Autodesk Fusion 360 part; units mm, degrees
sketch "Sketch4" plane through (0, 0, 0) normal (0, 0, 1) x (1, 0, 0)
  line L0 (53.2905, 24.45) -> (-53.2905, 24.45)
  line L1 (-53.2905, 24.45) -> (-53.2905, -24.45)
  line L2 (-53.2905, -24.45) -> (53.2905, -24.45)
  line L3 (53.2905, -24.45) -> (53.2905, 24.45)
  line L4 (53.2905, 24.45) -> (-53.2905, -24.45) construction
  line L5 (-53.2905, 24.45) -> (53.2905, -24.45) construction
  line L6 (-63.2905, -34.45) -> (63.2905, -34.45)
  line L7 (63.2905, -34.45) -> (63.2905, 34.45)
  line L8 (63.2905, 34.45) -> (-63.2905, 34.45)
  line L9 (-63.2905, 34.45) -> (-63.2905, -34.45)
  line L10 (-63.2905, -34.45) -> (63.2905, 34.45) construction
  line L11 (63.2905, -34.45) -> (-63.2905, 34.45) construction
  circle A0 centre (-58, 29) radius 1.45
  circle A1 centre (-58, -30) radius 1.45
  circle A2 centre (58.5, 29) radius 1.45
  circle A3 centre (58.5, -30) radius 1.45
  point P0 (-58, -30)
  dimension "d20" = 10
  dimension "d21" = 10
  dimension "d22" = 10
  dimension "d23" = 10
  dimension "d24" = 48.9
  dimension "d25" = 106.581
  dimension "d26" = 126.581
  dimension "d27" = 68.9
  dimension "d34" = 2.9
  dimension "d38" = 2.9
  dimension "d39" = 2.9
  dimension "d40" = 2.9
extrude "Extrude1" add sketch "Sketch4" along normal blind 3 contours L0 L1 L2 L3
extrude "Extrude2" add sketch "Sketch4" along normal blind 10
extrude "Extrude3" cut sketch "Sketch4" along normal blind 14 contours A0
extrude "Extrude4" cut sketch "Sketch4" along normal blind 14 contours A1
extrude "Extrude5" cut sketch "Sketch4" along normal blind 14 contours A3
extrude "Extrude6" cut sketch "Sketch4" along normal blind 14 contours A2
sketch "plate-2026-06-09T10_15_21.263Z" plane through (0, 0, 3) normal (0, 0, 1) x (1, 0, 0)
  line L0 (-24.2585, 6.9573) -> (-11.2585, 6.9573)
  line L1 (-24.2585, -7.0427) -> (-11.2585, -7.0427)
  line L2 (-24.7585, 6.4573) -> (-24.7585, -6.5427)
  line L3 (-10.7585, 6.4573) -> (-10.7585, -6.5427)
  arc A0 (-24.2585, 6.9573) -> (-24.7585, 6.4573) centre (-24.2585, 6.4573) ccw
  arc A1 (-10.7585, 6.4573) -> (-11.2585, 6.9573) centre (-11.2585, 6.4573) ccw
  arc A2 (-24.7585, -6.5427) -> (-24.2585, -7.0427) centre (-24.2585, -6.5427) ccw
  arc A3 (-11.2585, -7.0427) -> (-10.7585, -6.5427) centre (-11.2585, -6.5427) ccw
  line L4 (-5.2085, 6.9573) -> (7.7915, 6.9573)
  line L5 (-5.2085, -7.0427) -> (7.7915, -7.0427)
  line L6 (-5.7085, 6.4573) -> (-5.7085, -6.5427)
  line L7 (8.2915, 6.4573) -> (8.2915, -6.5427)
  arc A4 (-5.2085, 6.9573) -> (-5.7085, 6.4573) centre (-5.2085, 6.4573) ccw
  arc A5 (8.2915, 6.4573) -> (7.7915, 6.9573) centre (7.7915, 6.4573) ccw
  arc A6 (-5.7085, -6.5427) -> (-5.2085, -7.0427) centre (-5.2085, -6.5427) ccw
  arc A7 (7.7915, -7.0427) -> (8.2915, -6.5427) centre (7.7915, -6.5427) ccw
  line L8 (13.8415, 6.9573) -> (26.8415, 6.9573)
  line L9 (13.8415, -7.0427) -> (26.8415, -7.0427)
  line L10 (13.3415, 6.4573) -> (13.3415, -6.5427)
  line L11 (27.3415, 6.4573) -> (27.3415, -6.5427)
  arc A8 (13.8415, 6.9573) -> (13.3415, 6.4573) centre (13.8415, 6.4573) ccw
  arc A9 (27.3415, 6.4573) -> (26.8415, 6.9573) centre (26.8415, 6.4573) ccw
  arc A10 (13.3415, -6.5427) -> (13.8415, -7.0427) centre (13.8415, -6.5427) ccw
  arc A11 (26.8415, -7.0427) -> (27.3415, -6.5427) centre (26.8415, -6.5427) ccw
  line L12 (-53, -25) -> (53.2905, -24.45)
  line L13 (-53.2905, 24.45) -> (53.2905, 24.45)
  line L14 (-53, -25) -> (-53.2905, 24.45)
  line L15 (53.2905, -24.45) -> (53.2905, 24.45)
  line L16 (53.2905, -24.45) -> (53.2905, 24.45)
  line L17 (53.2905, 24.45) -> (-53.2905, 24.45)
  dimension "d65" = 13
  dimension "d66" = 13
  dimension "d67" = 13
  dimension "d68" = 13
  dimension "d69" = 13
  dimension "d70" = 13
  dimension "d71" = 49.45
  dimension "d72" = 106.2905
extrude "Extrude7" add sketch "plate-2026-06-09T10_15_21.263Z" along normal blind 3
extrude "Extrude8" cut sketch "plate-2026-06-09T10_15_21.263Z" along normal blind 3
Verification items for the finished model (mm, model axes). A direction names the side the tool comes from. Round coordinates to 2 decimals unless told otherwise and drop trailing zeros. Loops run counter-clockwise (first coordinate to the right, second up) from the corner with the lowest first, then second, coordinate; pieces in that order, holes last. Notation, with made-up numbers: (46.25, 35.5) - (99.25, 35.5) arc R27 ccw to (99.25, 59.5) - close; hole circle Ø1 at (-20, 43.5). An arc over 180 degrees is marked (long way). Answer in a Markdown table with one row per item. Add a question column.
Q1. Release check for a two-part mould opening along Z. For faces 3 (the face through (53.29, 0, 6)), 4 (the face through (-1, 0, 0)), 5 (the face through (-1, 31, 10)) record: pulls with the +Z half, pulls with the -Z half, needs draft (parallel to the pull), parting line crosses it, or undercut.
Q2. Section check B-B on y = -30. Enter the section's corners in (x, z).
Q3. Material ranges on line 1 (Y direction, x = -58, z = 5); line 2 (Y direction, x = 4.5, z = 7.25); line 3 (X direction, y = -20.5, z = 9), recorded low to high.
Q4. Section check D-D on x = -41.5. Enter the section's corners in (y, z), plus the area to 3 significant figures.
Q5. Section check C-C on y = -10.5. Enter the section's corners in (x, z), plus the area to 3 significant figures.
Q6. Section check A-A on x = 58.5. Enter the section's corners in (y, z).
Q7. Tool access check on faces 1 (the face through (-53.29, 0, 6)), 2 (the face through (-63.29, 0, 5)). Record the directions out of +Z, -Z, +X, -X, +Y, -Y that give a thin tool (end or side, any length) a straight path to the whole face; none if there is none.
Q8. Gauge pin test, flat end, axial feed: pin 1 (5 mm diameter, centred on x = -14, y = -8, fed in from -Z). Record the tip position at first contact, or that the pin passes through.
Found:
| question | item | result |
|---|---|---|
| 1 | face 3 | needs draft |
| 1 | face 4 | pulls with the -Z half |
| 1 | face 5 | pulls with the +Z half |
| 2 | outline | (-63.29, 0) - (-59.45, 0) - (-59.45, 10) - (-63.29, 10) - close; (-56.55, 0) - (57.05, 0) - (57.05, 10) - (-56.55, 10) - close; (59.95, 0) - (63.29, 0) - (63.29, 10) - (59.95, 10) - close |
| 3 | line 1 | y = -34.45 to -31.45, -28.55 to 27.55, 30.45 to 34.45 |
| 3 | line 2 | y = -34.45 to -24.45, 24.45 to 34.45 |
| 3 | line 3 | x = -63.29 to -53.29, 53.29 to 63.29 |
| 4 | outline | (-34.45, 0) - (34.45, 0) - (34.45, 10) - (24.45, 10) - (24.45, 3) - (-24.94, 3) - (-24.94, 6) - (-24.45, 6) - (-24.45, 10) - (-34.45, 10) - close |
| 4 | area | 345 mm² |
| 5 | outline | (-63.29, 0) - (63.29, 0) - (63.29, 10) - (53.29, 10) - (53.29, 3) - (-53.29, 3) - (-53.29, 10) - (-63.29, 10) - close |
| 5 | area | 520 mm² |
| 6 | outline | (-34.45, 0) - (-31.45, 0) - (-31.45, 10) - (-34.45, 10) - close; (-28.55, 0) - (27.55, 0) - (27.55, 10) - (-28.55, 10) - close; (30.45, 0) - (34.45, 0) - (34.45, 10) - (30.45, 10) - close |
| 7 | face 1 | +Z |
| 7 | face 2 | +Z, -Z, -X, +Y, -Y |
| 8 | pin 1 | stops at z = 0 |
